Geometry check sheet. Reference: the model listing, model coordinates, mm. A direction names the side the tool comes from. Round coordinates to 2 decimals unless told otherwise and drop trailing zeros. Order: outer loops, then holes, each group sorted by start corner. A loop starts at its lowest first (then second) coordinate and runs counter-clockwise, first axis right, second up.
(1) Thickness scan on L1, parallel to X at y = -92, z = 0.8; L2, parallel to X at y = -2, z = 0.75; L3, parallel to Y at x = 0, z = 1.2. Record the ranges inside material, lowest first.
(2) Cross-section at A-A on x = 0. Enter the section's corners in (y, z).
(3) Draft check along Y on faces 3 (the face through (-27.21, 28.76, 0.99)), 4 (the face through (31.127, 27.634, 0.986)), 5 (the face through (-1, -2, 2)). Enter one of: pulls with the +Y half, pulls with the -Y half, needs draft (parallel to the pull), parting line crosses it, or undercut.
(4) Cross-section at B-B on y = -45. Enter the section's corners in (x, z).
(5) Set-up check for faces 1 (the face through (-28.205, 25.182, 0.986)), 2 (the face through (27.24, 28.79, 0.99)): record each of +Z, -Z, +X, -X, +Y, -Y from which the full face is reachable in a straight line by a thin tool's end or side.
(6) Gauge pin test, flat ends, axial feed: P1, Ø1, axis at x = 5.5, z = 1, coming from the +Y side; P2, Ø4, axis at x = -23.17, y = 11.96, coming from the +Z side; P3, Ø1, axis at x = -18, z = 1.5, coming from the -Y side; P4, Ø0.6, axis at y = -94.5, z = 1, coming from the +X side. Record the tip position at first contact, or that the pin passes through.
(7) Cross-section at C-C on z = 0.55. Count the separate pieces of the cut face and the enclosed holes in it, and give its area (3 significant figures).
from build123d import *

# Parameters (mm, degrees)
SKETCH_3_R      = 2
SKETCH_3_R_2    = 1.999999995
SKETCH_3_R_3    = 1.5
SKETCH_3_R_4    = 33
EXTRUDE_1_DEPTH = 2


with BuildPart() as part:
    # 草图3 → 凸台-拉伸1 (new body)
    with BuildSketch(Plane.XY):
        with BuildLine():
            Line((-47, 31.317051182), (-47, -93.890216685))
            Line((-47, -93.890216685), (-45, -97.990216685))
            ThreePointArc((-45, -97.990216685), (-44.707106781, -98.697323466), (-44, -98.990216685))
            Line((-44, -98.990216685), (-25.9, -98.990216685))
            Line((-25.9, -98.990216685), (-25.9, -97.990216685))
            Line((-25.9, -97.990216685), (-25.9, -93.890216685))
            Line((-25.9, -93.890216685), (-15.9, -93.890216685))
            Line((-15.9, -93.890216685), (-6.948981504, -93.890216685))
            Line((-6.948981504, -93.890216685), (-6.948981504, -89.190216685))
            Line((-6.948981504, -89.190216685), (6.948981504, -89.190216685))
            Line((6.948981504, -89.190216685), (6.948981504, -93.890216685))
            Line((6.948981504, -93.890216685), (15.9, -93.890216685))
            Line((15.9, -93.890216685), (25.9, -93.890216685))
            Line((25.9, -93.890216685), (25.9, -97.990216685))
            Line((25.9, -97.990216685), (25.9, -98.990216685))
            Line((25.9, -98.990216685), (45, -98.990216685))
            Line((45, -98.990216685), (47, -93.890216685))
            Line((47, -93.890216685), (47, 31.317051182))
            Line((47, 31.317051182), (45, 31.317051182))
            ThreePointArc((45, 31.317051182), (36.482419799, 34.124770496), (28.474223712, 30.087289143))
            ThreePointArc((28.474223712, 30.087289143), (27.223611076, 28.776388924), (25.912710857, 27.525776288))
            ThreePointArc((25.912710857, 27.525776288), (15.928828372, 17.542283516), (1.809761925, 17.542559084))
            ThreePointArc((1.809761925, 17.542559084), (0, 17.5), (-1.809761925, 17.542559084))
            ThreePointArc((-1.809761925, 17.542559084), (-15.928828372, 17.542283516), (-25.912710857, 27.525776288))
            ThreePointArc((-25.912710857, 27.525776288), (-27.223611076, 28.776388924), (-28.474223712, 30.087289143))
            ThreePointArc((-28.474223712, 30.087289143), (-36.482419799, 34.124770496), (-45, 31.317051182))
            Line((-45, 31.317051182), (-47, 31.317051182))
        make_face()
        with Locations((0, 13.5)):
            Circle(SKETCH_3_R, mode=Mode.SUBTRACT)
        with Locations((-30.052038202, 25.947961669)):
            Circle(SKETCH_3_R_2, mode=Mode.SUBTRACT)
        with Locations((30.052038109, 25.947961893)):
            Circle(SKETCH_3_R_2, mode=Mode.SUBTRACT)
        with Locations((-23.174490752, 11.959783315)):
            Circle(SKETCH_3_R_3, mode=Mode.SUBTRACT)
        with Locations(Location((23.174490752, 11.959783315, 0), (0, 0, 180))):
            Circle(SKETCH_3_R_3, mode=Mode.SUBTRACT)
        with Locations((42.5, -14.940216685)):
            Circle(SKETCH_3_R_3, mode=Mode.SUBTRACT)
        with Locations(Location((-42.5, -14.940216685, 0), (0, 0, 180))):
            Circle(SKETCH_3_R_3, mode=Mode.SUBTRACT)
        with Locations((0, -39.340216685)):
            Circle(SKETCH_3_R_4, mode=Mode.SUBTRACT)
        with Locations((42.5, -84.940216685)):
            Circle(SKETCH_3_R_3, mode=Mode.SUBTRACT)
        with Locations((-42.5, -84.940216685)):
            Circle(SKETCH_3_R_3, mode=Mode.SUBTRACT)
        with BuildLine():
            Line((-37.1, -96.090216685), (-29.9, -96.090216685))
            Line((-29.9, -96.090216685), (-29.9, -93.890216685))
            Line((-29.9, -93.890216685), (-37.1, -93.890216685))
            ThreePointArc((-37.1, -93.890216685), (-37.555634919, -94.990216685), (-37.1, -96.090216685))
        make_face(mode=Mode.SUBTRACT)
        with BuildLine():
            Line((-43.6, -9.990216685), (-43.6, 25.009783315))
            ThreePointArc((-43.6, 25.009783315), (-42.5, 25.465418233), (-41.4, 25.009783315))
            Line((-41.4, 25.009783315), (-41.4, -9.990216685))
            ThreePointArc((-41.4, -9.990216685), (-42.5, -10.445851604), (-43.6, -9.990216685))
        make_face(mode=Mode.SUBTRACT)
        with BuildLine():
            Line((-41.4, -19.890216685), (-41.4, -25.190216685))
            Line((-41.4, -25.190216685), (-43.6, -25.190216685))
            Line((-43.6, -25.190216685), (-43.6, -19.890216685))
            ThreePointArc((-43.6, -19.890216685), (-42.5, -19.434581767), (-41.4, -19.890216685))
        make_face(mode=Mode.SUBTRACT)
        with BuildLine():
            Line((37.1, -93.890216685), (29.9, -93.890216685))
            Line((29.9, -93.890216685), (29.9, -96.090216685))
            Line((29.9, -96.090216685), (37.1, -96.090216685))
            ThreePointArc((37.1, -96.090216685), (37.555634919, -94.990216685), (37.1, -93.890216685))
        make_face(mode=Mode.SUBTRACT)
        with BuildLine():
            Line((43.6, -25.190216685), (43.6, -19.890216685))
            ThreePointArc((43.6, -19.890216685), (42.5, -19.434581767), (41.4, -19.890216685))
            Line((41.4, -19.890216685), (41.4, -25.190216685))
            Line((41.4, -25.190216685), (43.6, -25.190216685))
        make_face(mode=Mode.SUBTRACT)
        with BuildLine():
            Line((43.6, -95.190216685), (43.6, -89.890216685))
            ThreePointArc((43.6, -89.890216685), (42.5, -89.434581767), (41.4, -89.890216685))
            Line((41.4, -89.890216685), (41.4, -95.190216685))
            Line((41.4, -95.190216685), (43.6, -95.190216685))
        make_face(mode=Mode.SUBTRACT)
        with BuildLine():
            Line((41.4, -74.890216685), (41.4, -80.090216685))
            ThreePointArc((41.4, -80.090216685), (42.5, -80.545851604), (43.6, -80.090216685))
            Line((43.6, -80.090216685), (43.6, -74.890216685))
            Line((43.6, -74.890216685), (41.4, -74.890216685))
        make_face(mode=Mode.SUBTRACT)
        with BuildLine():
            Line((-41.4, -95.190216685), (-41.4, -89.890216685))
            ThreePointArc((-41.4, -89.890216685), (-42.5, -89.434581767), (-43.6, -89.890216685))
            Line((-43.6, -89.890216685), (-43.6, -95.190216685))
            Line((-43.6, -95.190216685), (-41.4, -95.190216685))
        make_face(mode=Mode.SUBTRACT)
        with BuildLine():
            Line((-43.6, -74.890216685), (-43.6, -80.090216685))
            ThreePointArc((-43.6, -80.090216685), (-42.5, -80.545851604), (-41.4, -80.090216685))
            Line((-41.4, -80.090216685), (-41.4, -74.890216685))
            Line((-41.4, -74.890216685), (-43.6, -74.890216685))
        make_face(mode=Mode.SUBTRACT)
        with BuildLine():
            Line((41.4, 25.009783315), (41.4, -9.990216685))
            ThreePointArc((41.4, -9.990216685), (42.5, -10.445851604), (43.6, -9.990216685))
            Line((43.6, -9.990216685), (43.6, 25.009783315))
            ThreePointArc((43.6, 25.009783315), (42.5, 25.465418233), (41.4, 25.009783315))
        make_face(mode=Mode.SUBTRACT)
    extrude(amount=EXTRUDE_1_DEPTH)


solid = part.part
Found:
1. L1: x = -47 to -43.6, -41.4 to -6.95, 6.95 to 41.4, 43.6 to 47
1. L2: x = -47 to -43.6, -41.4 to 41.4, 43.6 to 47
1. L3: y = -89.19 to -72.34, -6.34 to 11.5, 15.5 to 17.5
2. outline: (-89.19, 0) - (-72.34, 0) - (-72.34, 2) - (-89.19, 2) - close; (-6.34, 0) - (11.5, 0) - (11.5, 2) - (-6.34, 2) - close; (15.5, 0) - (17.5, 0) - (17.5, 2) - (15.5, 2) - close
3. face 3: pulls with the +Y half
3. face 4: undercut
3. face 5: needs draft
4. outline: (-47, 0) - (-32.51, 0) - (-32.51, 2) - (-47, 2) - close; (32.51, 0) - (47, 0) - (47, 2) - (32.51, 2) - close
5. face 1: +Z, -Z
5. face 2: +Z, -Z, +Y
6. P1: stops at y = 16.55
6. P2: stops at z = 2
6. P3: stops at y = -93.89
6. P4: stops at x = 46.88
7. separate pieces: 1
7. enclosed holes: 20
7. area: 7,520 mm2
